Source: CAD feature listing. Evaluate the final solid. Frame: model axes, mm. Face numbers are marked on the shaded views. A direction names the side the tool comes from. Round coordinates to 2 decimals unless told otherwise and drop trailing zeros. Order: outer loops, then holes, each group sorted by start corner. A loop starts at its lowest first (then second) coordinate and runs counter-clockwise, first axis right, second up. Notation, with made-up numbers: (78, -19.75) -> (98, -19.75) arc R6 ccw to (98, -11.75) -> close; hole circle Ø4 at (-17.75, 2). An arc over 180 degrees is marked (long way). Use a Markdown table: item, result. Add a question column.
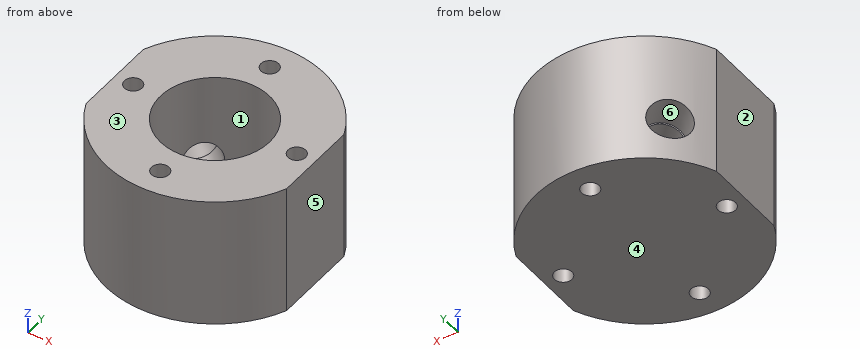
```python
from build123d import *

# Parameters (mm, degrees)
BOSS_EXTRUDE1_DEPTH    = 30
SKETCH6_R              = 12.5
CUT_EXTRUDE1_DEPTH     = 25
F_10_32_TAPPED_HOLE1_D = 4.0386


# Read off the part's stored shape, not the designer's step: 1/8 NPT Tapped Hole1
with BuildPart() as part:
    # Sketch2 → Boss-Extrude1 (new body)
    with BuildSketch(Plane.XY):
        with BuildLine():
            Line((-23, 9.797958971), (-23, -9.797958971))
            ThreePointArc((-23, -9.797958971), (0, -25), (23, -9.797958971))
            Line((23, -9.797958971), (23, 9.797958971))
            ThreePointArc((23, 9.797958971), (0, 25), (-23, 9.797958971))
        make_face()
    extrude(amount=BOSS_EXTRUDE1_DEPTH)

    # Sketch6 → Cut-Extrude1 (cut)
    with BuildSketch(Plane(origin=(0, 0, 30), x_dir=(-1, 0, 0), z_dir=(0, 0, 1))):
        with Locations(Location((0, 0, 0), (0, 0, 180))):
            Circle(SKETCH6_R)
    extrude(amount=-CUT_EXTRUDE1_DEPTH, mode=Mode.SUBTRACT)

    # #10-32 Tapped Hole1 (through all)
    with Locations(Plane.XY.offset(30)):
        with Locations((-18.75, 0), (0, 18.75), (18.75, 0), (0, -18.75)):
            Hole(F_10_32_TAPPED_HOLE1_D / 2)

    # 1/8 NPT Tapped Hole1 outline → 1/8 NPT Tapped Hole1 (revolve, cut)
    with BuildSketch(Plane(origin=(0, 0, 10), x_dir=(0.707106781186546, 0.707106781186549, 0), z_dir=(0, 0, -1))):
        Polygon((4.744600282, -25.000243213), (4.537398933, -18.08), (4.2164, -18.08), (4.2164, -11.766981388), (0, -11.766981388), (0, -25.000243213), align=None)
    revolve(axis=Axis((0, 0, 10), (0.707106781186549, -0.707106781186546, 0)), mode=Mode.SUBTRACT)


solid = part.part
```
1) Section C-C on z = 28. Output: boundary loops of the cut face in (x, y).
2) Section B-B on y = 0. Output: boundary loops of the cut face in (x, z), then the cut area to 3 significant figures.
3) Section A-A on x = 0. Output: boundary loops of the cut face in (y, z), then the cut area to 3 significant figures.
4) First-contact query: pin 1 Ø6.5 at (x, y) = (18.75, 0) entering from +Z; pin 2 Ø2 at (x, z) = (-17, 23) entering from +Y; pin 3 Ø3 at (x, z) = (17, 22) entering from +Y; pin 4 Ø8 at (x, z) = (8.5, 26.5) entering from +Y. Flat tips, straight axial feed; report the tip coordinate or a pass-through.
5) Section D-D on x = 18.75. Output: boundary loops of the cut face in (y, z).
6) Line query: probe 1 along X at (y, z) = (-4, 23); probe 2 along Y at (x, z) = (20.5, 1.5); probe 3 along X at (y, z) = (-18, 25). Output: solid intervals per line, ascending. Write a range as from..to.
7) Reachability of the marked faces 1 and 2 from +Z, -Z, +X, -X, +Y, -Y: full face, straight path, thin tool, end or side. Return the list, or none.
8) Draft query along Z for the marked faces 3, 4, 5 and 6. Return one class per face: pulls with the +Z half, pulls with the -Z half, needs draft (parallel to the pull), parting line crosses it, or undercut.
Conclusion:
| question | item | result |
|---|---|---|
| 1 | outline | (-23, -9.8) arc R25 ccw to (23, -9.8) -> (23, 9.8) arc R25 ccw to (-23, 9.8) -> close; hole circle Ø4.04 at (-18.75, 0); hole circle Ø25 at (0, 0); hole circle Ø4.04 at (0, -18.75); hole circle Ø4.04 at (0, 18.75); hole circle Ø4.04 at (18.75, 0) |
| 2 | outline | (-23, 0) -> (-20.77, 0) -> (-20.77, 30) -> (-23, 30) -> close; (-16.73, 0) -> (16.73, 0) -> (16.73, 30) -> (12.5, 30) -> (12.5, 5) -> (-12.5, 5) -> (-12.5, 30) -> (-16.73, 30) -> close; (20.77, 0) -> (23, 0) -> (23, 30) -> (20.77, 30) -> close |
| 2 | area | 513 mm^2 |
| 3 | outline | (-25, 0) -> (-20.77, 0) -> (-20.77, 30) -> (-25, 30) -> close; (-16.73, 0) -> (16.73, 0) -> (16.73, 30) -> (12.5, 30) -> (12.5, 5) -> (-12.5, 5) -> (-12.5, 30) -> (-16.73, 30) -> close; (20.77, 0) -> (25, 0) -> (25, 30) -> (20.77, 30) -> close |
| 3 | area | 633 mm^2 |
| 4 | pin 1 | stops at z = 30 |
| 4 | pin 2 | stops at y = 19.21 |
| 4 | pin 3 | stops at y = 19.62 |
| 4 | pin 4 | stops at y = 24.59 |
| 5 | outline | (-16.54, 0) -> (-2.02, 0) -> (-2.02, 30) -> (-16.54, 30) -> close; (2.02, 0) -> (16.54, 0) -> (16.54, 30) -> (2.02, 30) -> close |
| 6 | probe 1 | x = -23..-11.84, 11.84..23 |
| 6 | probe 2 | y = -14.31..-1.01, 1.01..14.31 |
| 6 | probe 3 | x = -17.35..-1.87, 1.87..17.35 |
| 7 | face 1 | +Z |
| 7 | face 2 | +Z, -Z, -X, +Y, -Y |
| 8 | face 3 | pulls with the +Z half |
| 8 | face 4 | pulls with the -Z half |
| 8 | face 5 | needs draft |
| 8 | face 6 | undercut |
